The listing builds one solid part. Answer for the finished solid, in the listing's coordinates (mm). A direction names the side the tool comes from. Coordinates: 2 decimals unless noted, no trailing zeros. Write each loop counter-clockwise with the first axis right and the second up, starting at its lowest first coordinate (ties: lowest second). Pieces come first, ordered by that corner, then holes.
from build123d import *

# Parameters (mm, degrees)
F1_DEPTH = 120


# Not quite as in the source:
# - ends of sketch curves that miss each other by under 0.0002 mm in the source are joined
# - the program builds the solid bodies; features that only make, move or delete a surface that nothing else refers to are left out


with BuildPart() as f1:
    # F0 (on Top) → F1 (new body)
    with BuildSketch(Plane.XY):
        with BuildLine():
            Line((3.939341, -5), (6.799995, -7.860656))
            Line((6.799995, -7.860656), (6.799995, -12.199997))
            ThreePointArc((6.799995, -12.199997), (6.7121307415, -12.4121300846), (6.5, -12.5))
            Line((6.5, -12.5), (4.599998, -12.5))
            ThreePointArc((4.599998, -12.5), (4.2464446094, -12.6464466094), (4.099998, -13))
            Line((4.099998, -13), (4.099998, -14.699997))
            ThreePointArc((4.099998, -14.699997), (4.1878632585, -14.9121300846), (4.399994, -15))
            Line((4.399994, -15), (12.5, -15))
            ThreePointArc((12.5, -15), (14.267766953, -14.267766953), (15, -12.5))
            Line((15, -12.5), (15, -4.399994))
            ThreePointArc((15, -4.399994), (14.9121300846, -4.1878632585), (14.699997, -4.099999))
            Line((14.699997, -4.099999), (13, -4.099998))
            ThreePointArc((13, -4.099998), (12.6464466094, -4.2464446094), (12.5, -4.599998))
            Line((12.5, -4.599998), (12.5, -6.5))
            ThreePointArc((12.5, -6.5), (12.4121300846, -6.7121307415), (12.199997, -6.799995))
            Line((12.199997, -6.799995), (7.860655, -6.799995))
            Line((7.860655, -6.799995), (5, -3.93934))
            Line((5, -3.93934), (5, 3.939341))
            Line((5, 3.939341), (7.860655, 6.799995))
            Line((7.860655, 6.799995), (12.199997, 6.799995))
            ThreePointArc((12.199997, 6.799995), (12.4121300846, 6.7121307415), (12.5, 6.5))
            Line((12.5, 6.5), (12.5, 4.599998))
            ThreePointArc((12.5, 4.599998), (12.6464466094, 4.2464446094), (13, 4.099998))
            Line((13, 4.099998), (14.699997, 4.099998))
            ThreePointArc((14.699997, 4.099998), (14.9121300846, 4.1878632585), (15, 4.399994))
            Line((15, 4.399994), (15, 12.5))
            ThreePointArc((15, 12.5), (14.267766953, 14.267766953), (12.5, 15))
            Line((12.5, 15), (4.399994, 15))
            ThreePointArc((4.399994, 15), (4.1878632585, 14.9121300846), (4.099999, 14.699997))
            Line((4.099999, 14.699997), (4.099998, 13))
            ThreePointArc((4.099998, 13), (4.2464446094, 12.6464466094), (4.599998, 12.5))
            Line((4.599998, 12.5), (6.5, 12.5))
            ThreePointArc((6.5, 12.5), (6.7121307415, 12.4121300846), (6.799995, 12.199997))
            Line((6.799995, 12.199997), (6.799995, 7.860655))
            Line((6.799995, 7.860655), (3.939341, 5))
            Line((3.939341, 5), (-3.93934, 5))
            Line((-3.93934, 5), (-6.799995, 7.860655))
            Line((-6.799995, 7.860655), (-6.799995, 12.199997))
            ThreePointArc((-6.799995, 12.199997), (-6.7121307415, 12.4121300846), (-6.5, 12.5))
            Line((-6.5, 12.5), (-4.599998, 12.5))
            ThreePointArc((-4.599998, 12.5), (-4.2464446094, 12.6464466094), (-4.099998, 13))
            Line((-4.099998, 13), (-4.099998, 14.699997))
            ThreePointArc((-4.099998, 14.699997), (-4.1878632585, 14.9121300846), (-4.399994, 15))
            Line((-4.399994, 15), (-12.5, 15))
            ThreePointArc((-12.5, 15), (-14.267766953, 14.267766953), (-15, 12.5))
            Line((-15, 12.5), (-15, 4.399994))
            ThreePointArc((-15, 4.399994), (-14.9121300846, 4.1878632585), (-14.699997, 4.099999))
            Line((-14.699997, 4.099999), (-13, 4.099998))
            ThreePointArc((-13, 4.099998), (-12.6464466094, 4.2464446094), (-12.5, 4.599998))
            Line((-12.5, 4.599998), (-12.5, 6.5))
            ThreePointArc((-12.5, 6.5), (-12.4121300846, 6.7121307415), (-12.199997, 6.799995))
            Line((-12.199997, 6.799995), (-7.860656, 6.799995))
            Line((-7.860656, 6.799995), (-5, 3.939341))
            Line((-5, 3.939341), (-5, -3.93934))
            Line((-5, -3.93934), (-7.860656, -6.799995))
            Line((-7.860656, -6.799995), (-12.199997, -6.799995))
            ThreePointArc((-12.199997, -6.799995), (-12.4121300846, -6.7121307415), (-12.5, -6.5))
            Line((-12.5, -6.5), (-12.5, -4.599998))
            ThreePointArc((-12.5, -4.599998), (-12.6464466094, -4.2464446094), (-13, -4.099998))
            Line((-13, -4.099998), (-14.699997, -4.099998))
            ThreePointArc((-14.699997, -4.099998), (-14.9121300846, -4.1878632585), (-15, -4.399994))
            Line((-15, -4.399994), (-15, -12.5))
            ThreePointArc((-15, -12.5), (-14.267766953, -14.267766953), (-12.5, -15))
            Line((-12.5, -15), (-4.399994, -15))
            ThreePointArc((-4.399994, -15), (-4.1878632585, -14.9121300846), (-4.099999, -14.699997))
            Line((-4.099999, -14.699997), (-4.099998, -13))
            ThreePointArc((-4.099998, -13), (-4.2464446094, -12.6464466094), (-4.599998, -12.5))
            Line((-4.599998, -12.5), (-6.5, -12.5))
            ThreePointArc((-6.5, -12.5), (-6.7121307415, -12.4121300846), (-6.799995, -12.199997))
            Line((-6.799995, -12.199997), (-6.799995, -7.860656))
            Line((-6.799995, -7.860656), (-3.93934, -5))
            Line((-3.93934, -5), (3.939341, -5))
        make_face()
        with BuildLine():
            Line((-8.299995, -14), (-12.5, -14))
            ThreePointArc((-12.5, -14), (-13.5606601718, -13.5606601718), (-14, -12.5))
            Line((-14, -12.5), (-14, -8.299995))
            ThreePointArc((-14, -8.299995), (-13.8535533906, -7.9464416094), (-13.5, -7.799995))
            Line((-13.5, -7.799995), (-9.299995, -7.799995))
            ThreePointArc((-9.299995, -7.799995), (-8.2393348282, -8.2393348282), (-7.799995, -9.299995))
            Line((-7.799995, -9.299995), (-7.799995, -13.5))
            ThreePointArc((-7.799995, -13.5), (-7.9464416094, -13.8535533906), (-8.299995, -14))
        make_face(mode=Mode.SUBTRACT)
        with BuildLine():
            Line((12.5, -14), (8.299995, -14))
            ThreePointArc((8.299995, -14), (7.9464416094, -13.8535533906), (7.799995, -13.5))
            Line((7.799995, -13.5), (7.799995, -9.299995))
            ThreePointArc((7.799995, -9.299995), (8.2393348282, -8.2393348282), (9.299995, -7.799995))
            Line((9.299995, -7.799995), (13.5, -7.799995))
            ThreePointArc((13.5, -7.799995), (13.8535533906, -7.9464416094), (14, -8.299995))
            Line((14, -8.299995), (14, -12.5))
            ThreePointArc((14, -12.5), (13.5606601718, -13.5606601718), (12.5, -14))
        make_face(mode=Mode.SUBTRACT)
        with BuildLine():
            Line((3.657288, -2.243073), (3.878887, -3.285876))
            ThreePointArc((3.878887, -3.285876), (3.7433613906, -3.7433613906), (3.2858769836, -3.8788870773))
            Line((3.2858769836, -3.8788870773), (2.243074, -3.657287))
            Line((2.243074, -3.657287), (2.005135, -3.419348))
            ThreePointArc((2.005135, -3.419348), (1.841799908, -3.3354753308), (1.6601868142, -3.3624816237))
            ThreePointArc((1.6601868142, -3.3624816237), (0, -3.75), (-1.6601870383, -3.3624810777))
            ThreePointArc((-1.6601870383, -3.3624810777), (-1.841799908, -3.3354753308), (-2.0051340344, -3.4193479656))
            Line((-2.0051340344, -3.4193479656), (-2.243073, -3.657287))
            Line((-2.243073, -3.657287), (-3.285876, -3.878887))
            ThreePointArc((-3.285876, -3.878887), (-3.7433613906, -3.7433613906), (-3.8788870773, -3.2858769836))
            Line((-3.8788870773, -3.2858769836), (-3.657287, -2.243073))
            Line((-3.657287, -2.243073), (-3.419348, -2.005134))
            ThreePointArc((-3.419348, -2.005134), (-3.3354753308, -1.841799908), (-3.3624816237, -1.6601868142))
            ThreePointArc((-3.3624816237, -1.6601868142), (-3.75, 0), (-3.3624810777, 1.6601870383))
            ThreePointArc((-3.3624810777, 1.6601870383), (-3.3354753883, 1.8418002569), (-3.4193484656, 2.0051345344))
            Line((-3.4193484656, 2.0051345344), (-3.657287, 2.243074))
            Line((-3.657287, 2.243074), (-3.878887, 3.285877))
            ThreePointArc((-3.878887, 3.285877), (-3.7433613906, 3.7433613906), (-3.2858769836, 3.8788870773))
            Line((-3.2858769836, 3.8788870773), (-2.243073, 3.657288))
            Line((-2.243073, 3.657288), (-2.005134, 3.419348))
            ThreePointArc((-2.005134, 3.419348), (-1.8418001264, 3.3354753668), (-1.6601872112, 3.3624814277))
            ThreePointArc((-1.6601872112, 3.3624814277), (0, 3.75), (1.6601870383, 3.3624810777))
            ThreePointArc((1.6601870383, 3.3624810777), (1.8418002569, 3.3354753883), (2.0051345344, 3.4193484656))
            Line((2.0051345344, 3.4193484656), (2.243074, 3.657288))
            Line((2.243074, 3.657288), (3.285877, 3.878887))
            ThreePointArc((3.285877, 3.878887), (3.7433610448, 3.7433617364), (3.8788872806, 3.2858779404))
            Line((3.8788872806, 3.2858779404), (3.657288, 2.243074))
            Line((3.657288, 2.243074), (3.419348, 2.005135))
            ThreePointArc((3.419348, 2.005135), (3.3354753668, 1.8418001264), (3.3624814277, 1.6601872112))
            ThreePointArc((3.3624814277, 1.6601872112), (3.75, 0), (3.3624810777, -1.6601870383))
            ThreePointArc((3.3624810777, -1.6601870383), (3.3354753308, -1.841799908), (3.4193479656, -2.0051340344))
            Line((3.4193479656, -2.0051340344), (3.657288, -2.243073))
        make_face(mode=Mode.SUBTRACT)
        with BuildLine():
            Line((-9.299995, 7.799995), (-13.5, 7.799995))
            ThreePointArc((-13.5, 7.799995), (-13.8535533906, 7.9464416094), (-14, 8.299995))
            Line((-14, 8.299995), (-14, 12.5))
            ThreePointArc((-14, 12.5), (-13.5606601718, 13.5606601718), (-12.5, 14))
            Line((-12.5, 14), (-8.299995, 14))
            ThreePointArc((-8.299995, 14), (-7.9464416094, 13.8535533906), (-7.799995, 13.5))
            Line((-7.799995, 13.5), (-7.799995, 9.299995))
            ThreePointArc((-7.799995, 9.299995), (-8.2393348282, 8.2393348282), (-9.299995, 7.799995))
        make_face(mode=Mode.SUBTRACT)
        with BuildLine():
            Line((13.5, 7.799995), (9.299995, 7.799995))
            ThreePointArc((9.299995, 7.799995), (8.2393348282, 8.2393348282), (7.799995, 9.299995))
            Line((7.799995, 9.299995), (7.799995, 13.5))
            ThreePointArc((7.799995, 13.5), (7.9464416094, 13.8535533906), (8.299995, 14))
            Line((8.299995, 14), (12.5, 14))
            ThreePointArc((12.5, 14), (13.5606601718, 13.5606601718), (14, 12.5))
            Line((14, 12.5), (14, 8.299995))
            ThreePointArc((14, 8.299995), (13.8535533906, 7.9464416094), (13.5, 7.799995))
        make_face(mode=Mode.SUBTRACT)
    extrude(amount=F1_DEPTH)


solid = f1.part
Q1. The part is cut by section B-B, the plane z = 109. State how many separate pieces and enclosed holes the cut face has, then the cut area to 3 significant figures.
Answers below:
separate pieces: 1
enclosed holes: 5
area: 234 mm2
Q2. Determine the mould class of faces 6 (the face through (-6.45, 5.39, 59.16)), 7 (the face through (-5, 0, 59)), 8 (the face through (15, -9, 59)) for opening direction X: released by +X, released by -X, zero draft, split by the parting line, or undercut.
Answers below:
face 6: undercut
face 7: released by -X
face 8: released by +X
Q3. Given pin 1 (10 mm diameter, centred on x = 0.5, y = -8, fed in from +Z); pin 2 (1.4 mm diameter, centred on y = 14, z = 43, fed in from -X); pin 3 (0.8 mm diameter, centred on x = 14, z = 32, fed in from -Y) (3 decimals); pin 4 (0.5 mm diameter, centred on y = -14, z = 49, fed in from -X), each flat-ended and moving along its own axis, determine where each tip first touches the part or whether it passes through.
Answers below:
pin 1: stops at z = 120
pin 2: stops at x = -14.87
pin 3: stops at y = -14.745
pin 4: stops at x = -14.67
Q4. Find the intervals of material crossed by probe 1 along Y at (x, z) = (-12, 107.5); probe 2 along X at (y, z) = (-13.25, 71), in increasing order.
Answers below:
probe 1: y = -15 to -14, -7.8 to -6.8, 6.8 to 7.8, 14 to 15
probe 2: x = -14.88 to -13.8, -7.8 to -4.1, 4.1 to 7.8, 13.8 to 14.88
Q5. The part is cut by section A-A, the plane y = 10.75. Write down the section's boundary in (x, z).
Answers below:
outline: (-15, 0) - (-14, 0) - (-14, 120) - (-15, 120) - close; (-7.8, 0) - (-6.8, 0) - (-6.8, 120) - (-7.8, 120) - close; (6.8, 0) - (7.8, 0) - (7.8, 120) - (6.8, 120) - close; (14, 0) - (15, 0) - (15, 120) - (14, 120) - close
Q6. Which of the six approach directions +Z, -Z, +X, -X, +Y, -Y give full straight-line access (tool end or side, diameter ignored) to faces 1 (the face through (-14.248, 14.287, 59.16)), 2 (the face through (0, -5, 59)), 3 (the face through (10, 6.8, 59)), 4 (the face through (8, -15, 59)), 5 (the face through (5, 0, 59))?
Answers below:
face 1: +Z, -Z, -X, +Y
face 2: +Z, -Z, -Y
face 3: +Z, -Z
face 4: +Z, -Z, +X, -X, -Y
face 5: +Z, -Z, +X
